Can you work these out from the drawing? Everything is in mm from the part's minimum corner. A direction names the side the tool comes from. Round coordinates to 2 decimals unless told otherwise and drop trailing zeros. Write each loop counter-clockwise with the first axis right and the second up, starting at its lowest first coordinate (ties: lowest second). Pieces come first, ordered by that corner, then holes. Notation, with made-up numbers: (-22, 86) - (10, 86) arc R26 cw to (10, 120) - close; hole circle Ø8 at (-15, 72). An arc over 180 degrees is marked (long way). One line per item, written item: value. Start each with the question number.
Item 1: For the marked faces 1 and 2, which set-ups out of +Z, -Z, +X, -X, +Y, -Y let a thin tool reach every point of the face, with its end or its side?
Item 2: Imagine slicing it at B-B, the plane x = 6. Please give me the cut outline in (y, z).
Item 3: For P1, Ø10, axis at y = 25, z = 10.5, coming from the -X side; P2, Ø8, axis at x = 9.5, y = 8.5, coming from the +Z side; P3, Ø10, axis at x = 3.5, z = 14.5, coming from the -Y side, each with a flat end and sliding along its axis, tell me the tip position at first contact or that it passes through.
Item 4: If I drill on line 1 (Y direction, x = 20, z = 1.7); line 2 (Z direction, x = 15.5, y = 29); line 3 (Y direction, x = 8.75, z = 13.75), over which ranges is the centre line in solid material (lowest first)?
Item 5: Imagine slicing it at C-C, the plane z = 8.5. Please give me the cut outline in (x, y).
Item 6: Imagine slicing it at D-D, the plane x = 17.5. Please give me the cut outline in (y, z), then the cut area to 3 significant figures.
Item 7: Imagine slicing it at A-A, the plane y = 7. Please give me the cut outline in (x, z).
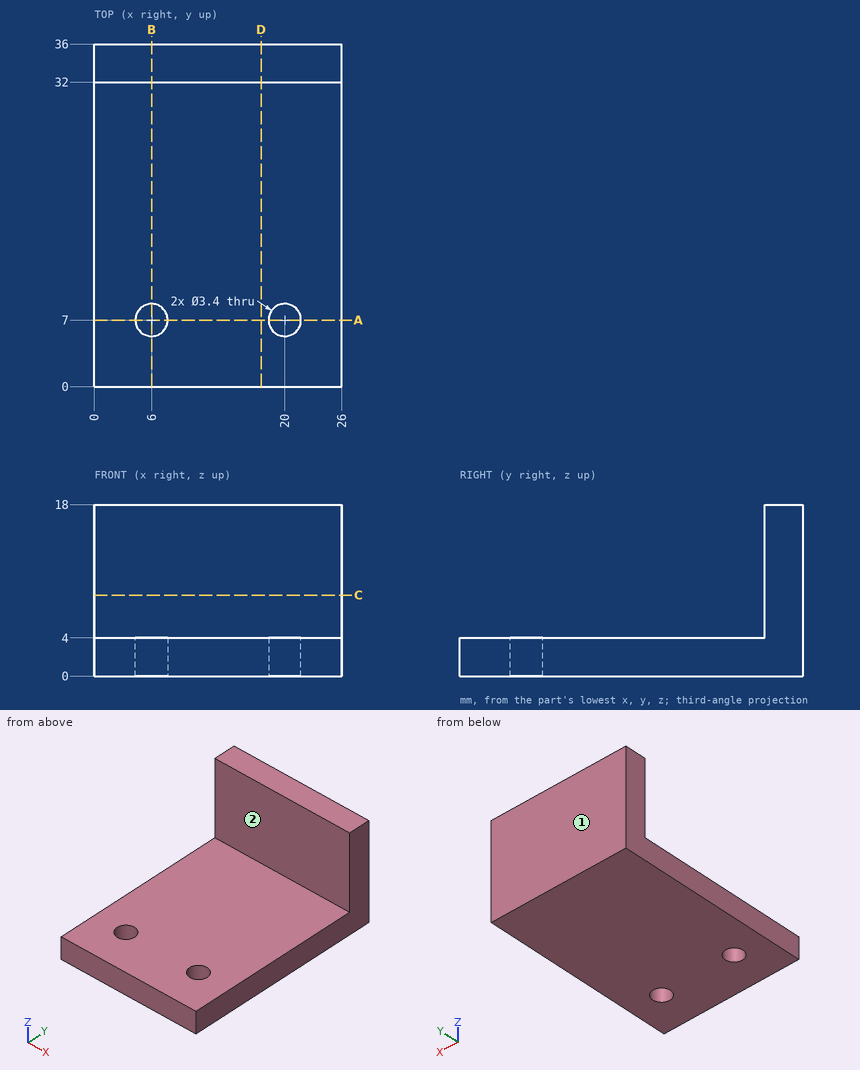
Values follow:
1. face 1: +Z, -Z, +X, -X, +Y
1. face 2: +Z, +X, -X, -Y
2. outline: (0, 0) - (5.3, 0) - (5.3, 4) - (0, 4) - close; (8.7, 0) - (36, 0) - (36, 18) - (32, 18) - (32, 4) - (8.7, 4) - close
3. P1: passes through
3. P2: stops at z = 4
3. P3: stops at y = 32
4. line 1: y = 0 to 5.3, 8.7 to 36
4. line 2: z = 0 to 4
4. line 3: y = 32 to 36
5. outline: (0, 32) - (26, 32) - (26, 36) - (0, 36) - close
6. outline: (0, 0) - (36, 0) - (36, 18) - (32, 18) - (32, 4) - (0, 4) - close
6. area: 200 mm^2
7. outline: (0, 0) - (4.3, 0) - (4.3, 4) - (0, 4) - close; (7.7, 0) - (18.3, 0) - (18.3, 4) - (7.7, 4) - close; (21.7, 0) - (26, 0) - (26, 4) - (21.7, 4) - close
